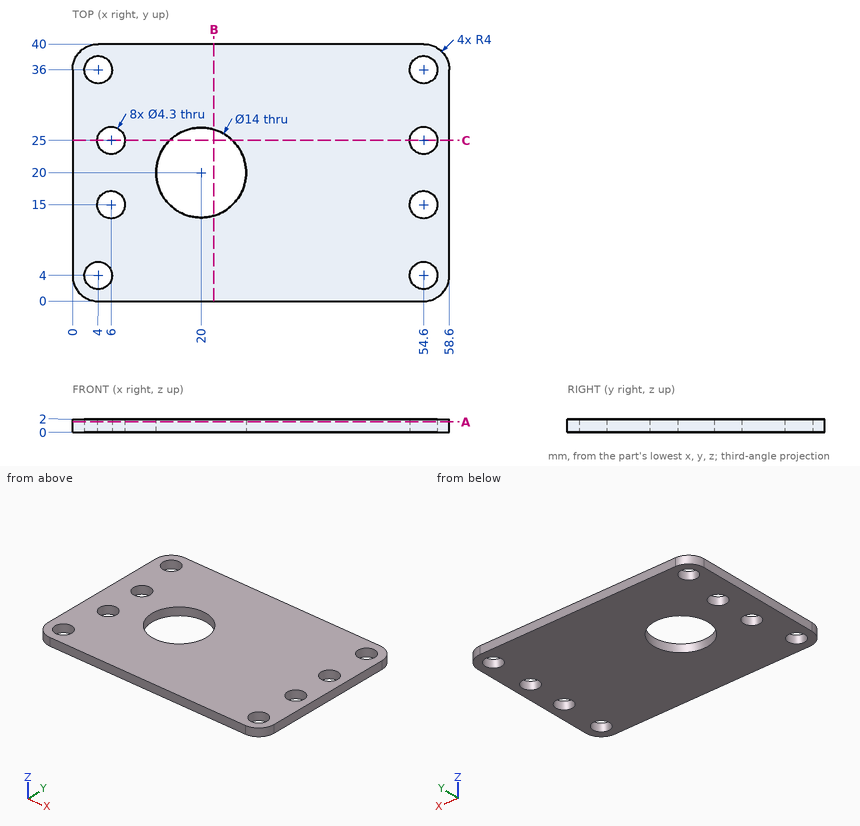
Verification items for this drawing (mm, ordinates from the low corner). Coordinates: 2 decimals unless noted, no trailing zeros. Write each loop counter-clockwise with the first axis right and the second up, starting at its lowest first coordinate (ties: lowest second). Pieces come first, ordered by that corner, then holes. Notation, with made-up numbers: M 35.25,13 L 45.25,13 A35 ccw 45.25,48 Z; hole C 68.25,51.5 d9. An arc over 180 degrees is marked long. Answer as a JSON object with one key per item and string values.
1. Section check B-B, the plane x = 22. Enter the section's corners in (y, z).
Answers below:
{"outline": "M 0,0 L 13.29,0 L 13.29,2 L 0,2 Z; M 26.71,0 L 40,0 L 40,2 L 26.71,2 Z"}
2. Scan lines: L1, parallel to Y at x = 54.6, z = 0.65; L2, parallel to X at y = 20, z = 0.5; L3, parallel to X at y = 15, z = 0.65. Record each from-to range of solid material in increasing order.
Answers below:
{"L1": "y = 0 to 1.85, 6.15 to 12.85, 17.15 to 22.85, 27.15 to 33.85, 38.15 to 40", "L2": "x = 0 to 13, 27 to 58.6", "L3": "x = 0 to 3.85, 8.15 to 15.1, 24.9 to 52.45, 56.75 to 58.6"}
3. Section check C-C, the plane y = 25. Enter the section's corners in (x, z), plus the area to 3 significant figures.
Answers below:
{"outline": "M 0,0 L 3.85,0 L 3.85,2 L 0,2 Z; M 8.15,0 L 15.1,0 L 15.1,2 L 8.15,2 Z; M 24.9,0 L 52.45,0 L 52.45,2 L 24.9,2 Z; M 56.75,0 L 58.6,0 L 58.6,2 L 56.75,2 Z", "area": "80.4 mm²"}
4. Section check A-A, the plane z = 1.6. Give the number of separate pieces and of enclosed holes in the cut face, plus the area to 3 significant figures.
Answers below:
{"separate pieces": "1", "enclosed holes": "9", "area": "2,060 mm²"}
